from build123d import *

# Parameters (mm, degrees)
BOSS_EXTRUDE1_DEPTH              = 1.6
BOSS_EXTRUDE2_DEPTH              = 0.1
M1_6_HOLE1_FIXINGSTRUCTURE_D     = 1.8
M1_6_HOLE1_FIXINGSTRUCTURE_DEPTH = 200
M1_6_HOLE1_FIXINGSTRUCTURE_TIP   = 0.540774557


with BuildPart() as part:
    # Sketch1 → Boss-Extrude1 (new body)
    with BuildSketch(Plane.XY):
        with BuildLine():
            Line((-34, 44), (-34, 38))
            ThreePointArc((-34, 38), (-34.146446609, 37.646446609), (-34.5, 37.5))
            Line((-34.5, 37.5), (-40.5, 37.5))
            ThreePointArc((-40.5, 37.5), (-40.853553391, 37.353553391), (-41, 37))
            Line((-41, 37), (-41, -37))
            ThreePointArc((-41, -37), (-40.853553391, -37.353553391), (-40.5, -37.5))
            Line((-40.5, -37.5), (-34.5, -37.5))
            ThreePointArc((-34.5, -37.5), (-34.146446609, -37.646446609), (-34, -38))
            Line((-34, -38), (-34, -44))
            ThreePointArc((-34, -44), (-33.853553391, -44.353553391), (-33.5, -44.5))
            Line((-33.5, -44.5), (33.5, -44.5))
            ThreePointArc((33.5, -44.5), (33.853553391, -44.353553391), (34, -44))
            Line((34, -44), (34, -38))
            ThreePointArc((34, -38), (34.146446609, -37.646446609), (34.5, -37.5))
            Line((34.5, -37.5), (40.5, -37.5))
            ThreePointArc((40.5, -37.5), (40.853553391, -37.353553391), (41, -37))
            Line((41, -37), (41, 37))
            ThreePointArc((41, 37), (40.853553391, 37.353553391), (40.5, 37.5))
            Line((40.5, 37.5), (34.5, 37.5))
            ThreePointArc((34.5, 37.5), (34.146446609, 37.646446609), (34, 38))
            Line((34, 38), (34, 44))
            ThreePointArc((34, 44), (33.853553391, 44.353553391), (33.5, 44.5))
            Line((33.5, 44.5), (-33.5, 44.5))
            ThreePointArc((-33.5, 44.5), (-33.853553391, 44.353553391), (-34, 44))
        make_face()
    extrude(amount=BOSS_EXTRUDE1_DEPTH)

    # Esboço1 → Boss-Extrude2 (add)
    with BuildSketch(Plane.XY.offset(1.6)):
        with BuildLine():
            Line((-29.5, -37.5), (29.5, -37.5))
            ThreePointArc((29.5, -37.5), (33.035533906, -36.035533906), (34.5, -32.5))
            Line((34.5, -32.5), (34.5, 32.5))
            ThreePointArc((34.5, 32.5), (33.035533906, 36.035533906), (29.5, 37.5))
            Line((29.5, 37.5), (-29.5, 37.5))
            ThreePointArc((-29.5, 37.5), (-33.035533906, 36.035533906), (-34.5, 32.5))
            Line((-34.5, 32.5), (-34.5, -32.5))
            ThreePointArc((-34.5, -32.5), (-33.035533906, -36.035533906), (-29.5, -37.5))
        make_face()
    extrude(amount=BOSS_EXTRUDE2_DEPTH)

    # M1.6 Hole1-FixingStructure
    with Locations(Plane(origin=(0, 0, 0), x_dir=(-1, 0, 0), z_dir=(0, 0, -1))):
        with Locations((-30.5, 40.5), (30.5, 40.5), (-30.5, -40.5), (30.5, -40.5)):
            Hole(M1_6_HOLE1_FIXINGSTRUCTURE_D / 2, depth=M1_6_HOLE1_FIXINGSTRUCTURE_DEPTH)
            with Locations((0, 0, -(M1_6_HOLE1_FIXINGSTRUCTURE_DEPTH + M1_6_HOLE1_FIXINGSTRUCTURE_TIP / 2))):  # 118° drill point
                Cone(0, M1_6_HOLE1_FIXINGSTRUCTURE_D / 2, M1_6_HOLE1_FIXINGSTRUCTURE_TIP, mode=Mode.SUBTRACT)


solid = part.part
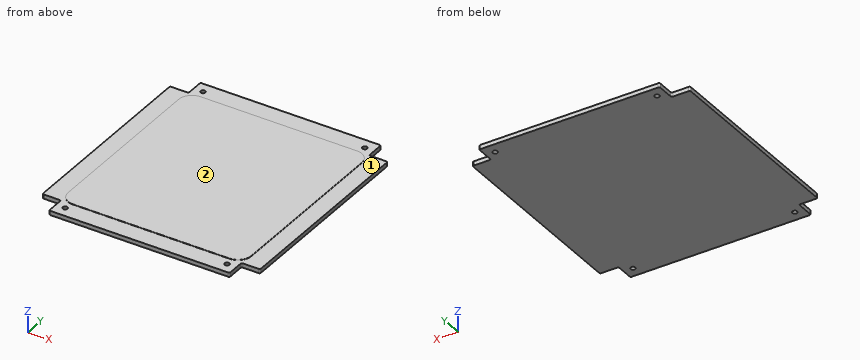
CAD build for the part. Positions are in the model's coordinates, mm. Face numbers are marked on the shaded views. A direction names the side the tool comes from. Give positions to 0.01 mm unless a question says otherwise; leave off trailing zeros. Order: outer loops, then holes, each group sorted by start corner. A loop starts at its lowest first (then second) coordinate and runs counter-clockwise, first axis right, second up. Notation, with made-up numbers: (36.25, -1) -> (42.25, -1) arc R14 ccw to (42.25, 16) -> close; hole circle Ø4 at (13.25, 13). An arc over 180 degrees is marked (long way). Return JSON: item names as keys, results as strings.
Q1. Which spindle directions (+Z, -Z, +X, -X, +Y, -Y) get a long thin tool onto all of the face, cutting with end or side? Do the marked faces 1 and 2. Say none if no direction does.
Working result:
{"face 1": "+Z", "face 2": "+Z, +X, -X, +Y, -Y"}
Q2. Drill centre lines: line 1 (Y direction, x = 30.5, z = 0.4); line 2 (X direction, y = -40.5, z = 1); line 3 (X direction, y = -40, z = 1.45). Where is each one in solid material? Low to high.
Working result:
{"line 1": "-44.5 to -41.4, -39.6 to 39.6, 41.4 to 44.5", "line 2": "-34 to -31.4, -29.6 to 29.6, 31.4 to 34", "line 3": "-34 to -31.25, -29.75 to 29.75, 31.25 to 34"}
Q3. Saw through at A-A (z = 0.3). Write the cut outline in (x, y).
Working result:
{"outline": "(-41, -37) arc R0.5 ccw to (-40.5, -37.5) -> (-34.5, -37.5) arc R0.5 cw to (-34, -38) -> (-34, -44) arc R0.5 ccw to (-33.5, -44.5) -> (33.5, -44.5) arc R0.5 ccw to (34, -44) -> (34, -38) arc R0.5 cw to (34.5, -37.5) -> (40.5, -37.5) arc R0.5 ccw to (41, -37) -> (41, 37) arc R0.5 ccw to (40.5, 37.5) -> (34.5, 37.5) arc R0.5 cw to (34, 38) -> (34, 44) arc R0.5 ccw to (33.5, 44.5) -> (-33.5, 44.5) arc R0.5 ccw to (-34, 44) -> (-34, 38) arc R0.5 cw to (-34.5, 37.5) -> (-40.5, 37.5) arc R0.5 ccw to (-41, 37) -> close; hole circle Ø1.8 at (-30.5, -40.5); hole circle Ø1.8 at (-30.5, 40.5); hole circle Ø1.8 at (30.5, -40.5); hole circle Ø1.8 at (30.5, 40.5)"}
Q4. Flat gauge pins, fed straight in: pin 1 (0.5 mm diameter, centred on y = 41, z = 0.5, fed in from +X); pin 2 (8 mm diameter, centred on x = -27, y = -24.5, fed in from -Z); pin 3 (1.4 mm diameter, centred on x = -30.5, y = 40.5, fed in from +Z); pin 4 (0.5 mm diameter, centred on x = -37.5, z = 1, fed in from -Y). Where does each tip first touch, or does it go through?
Working result:
{"pin 1": "x = 34", "pin 2": "z = 0", "pin 3": "through", "pin 4": "y = -37.5"}
